Verification items for this drawing (mm, ordinates from the low corner). A direction names the side the tool comes from. Give positions to 0.01 mm unless a question says otherwise; leave off trailing zeros. Loops run counter-clockwise (first coordinate to the right, second up) from the corner with the lowest first, then second, coordinate; pieces in that order, holes last. Notation, with made-up numbers: M 49,41.25 L 77,41.25 A35 ccw 77,79.25 Z; hole C 81.5,16 d1. An arc over 180 degrees is marked long. Use a Markdown table: item, result.
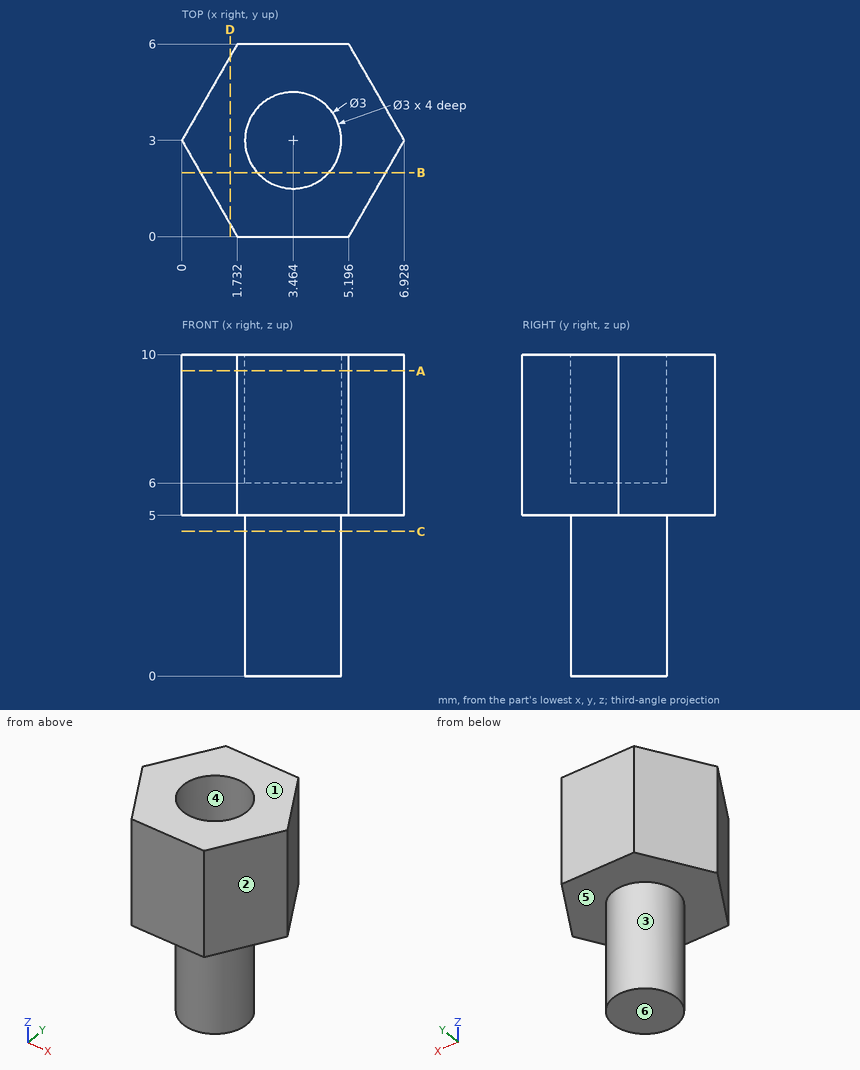
(1) Cross-section at C-C on z = 4.5. Record the cut outline in (x, y).
Results below:
| item | result |
|---|---|
| outline | C 3.46,3 d3 |
(2) Material ranges on line 1 (Y direction, x = 3.5, z = 6.75); line 2 (Z direction, x = 3.25, y = 0.75); line 3 (Y direction, x = 2.5, z = 9.25), recorded low to high.
Results below:
| item | result |
|---|---|
| line 1 | 0 to 1.5, 4.5 to 6 |
| line 2 | 5 to 10 |
| line 3 | 0 to 1.85, 4.15 to 6 |
(3) Draft check along Y on the marked faces 1, 2, 3 and 4. Enter one of: +Y half, -Y half, draft (parallel to the pull), parting line (faces both ways), or undercut.
Results below:
| item | result |
|---|---|
| face 1 | draft |
| face 2 | -Y half |
| face 3 | parting line |
| face 4 | undercut |
(4) Cross-section at B-B on y = 2. Record the cut outline in (x, z).
Results below:
| item | result |
|---|---|
| outline | M 0.58,5 L 2.35,5 L 2.35,0 L 4.58,0 L 4.58,5 L 6.35,5 L 6.35,10 L 4.58,10 L 4.58,6 L 2.35,6 L 2.35,10 L 0.58,10 Z |
(5) Cross-section at D-D on x = 1.5. Record the cut outline in (y, z).
Results below:
| item | result |
|---|---|
| outline | M 0.4,5 L 5.6,5 L 5.6,10 L 0.4,10 Z |
(6) Cross-section at A-A on z = 9.5. Record the cut outline in (x, y), then the cut area to 3 significant figures.
Results below:
| item | result |
|---|---|
| outline | M 0,3 L 1.73,0 L 5.2,0 L 6.93,3 L 5.2,6 L 1.73,6 Z; hole C 3.46,3 d3 |
| area | 24.1 mm^2 |
(7) Set-up check for the marked faces 5 and 6: record each of +Z, -Z, +X, -X, +Y, -Y from which the full face is reachable in a straight line by a thin tool's end or side.
Results below:
| item | result |
|---|---|
| face 5 | -Z |
| face 6 | -Z, +X, -X, +Y, -Y |
(8) Gauge pin test, flat ends, axial feed: P1, Ø2, axis at y = 5.5, z = 5.5, coming from the -X side; P2, Ø1.5, axis at y = 1, z = 1, coming from the -X side (1 decimal). Record the tip position at first contact, or that the pin passes through.
Results below:
| item | result |
|---|---|
| P1 | x = 0.87 |
| P2 | x = 2.6 |
